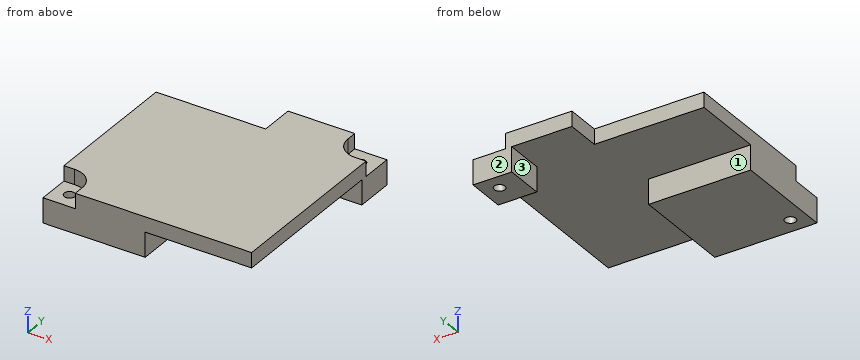
```python
from build123d import *

# Parameters (mm, degrees)
BOSS_EXTRUDE2_DEPTH     = 1.4
SKETCH2_W               = 3.6
SKETCH2_H               = 3.6
SKETCH2_W_2             = 9.5
SKETCH2_H_2             = 9.5
BOSS_EXTRUDE3_DEPTH     = 2.3
CUT_EXTRUDE1_DEPTH      = 14.909349374
CUT_EXTRUDE1_DEPTH_BACK = 14.909349374
SKETCH4_R               = 0.5


with BuildPart() as part:
    # Sketch1 → Boss-Extrude2 (new body)
    with BuildSketch(Plane.XY):
        with BuildLine():
            Line((-6.7, -9.7), (9.7, -9.7))
            Line((9.7, -9.7), (9.7, 6.7))
            Line((9.7, 6.7), (8.7, 6.7))
            ThreePointArc((8.7, 6.7), (7.285786438, 7.285786438), (6.7, 8.7))
            Line((6.7, 8.7), (6.7, 9.7))
            Line((6.7, 9.7), (0.5, 9.7))
            Line((0.5, 9.7), (0.5, 6.5))
            Line((0.5, 6.5), (-9.7, 6.5))
            Line((-9.7, 6.5), (-9.7, -6.7))
            Line((-9.7, -6.7), (-8.7, -6.7))
            ThreePointArc((-8.7, -6.7), (-7.285786438, -7.285786438), (-6.7, -8.7))
            Line((-6.7, -8.7), (-6.7, -9.7))
        make_face()
    extrude(amount=BOSS_EXTRUDE2_DEPTH)

    # Sketch2 → Boss-Extrude3 (add)
    with BuildSketch(Plane(origin=(0, 0, 0), x_dir=(-1, 0, 0), z_dir=(0, 0, -1))):
        with Locations((-7.9, 7.9)):
            Rectangle(SKETCH2_W, SKETCH2_H)
        with Locations((4.95, -4.95)):
            Rectangle(SKETCH2_W_2, SKETCH2_H_2)
    extrude(amount=BOSS_EXTRUDE3_DEPTH)

    # Sketch4 → Cut-Extrude1 (cut, two sides: drawn at the far end of the back side and taken through both)
    with BuildSketch(Plane.XY.offset(-CUT_EXTRUDE1_DEPTH_BACK)):
        with Locations((8.2, 8.2)):
            Circle(SKETCH4_R)
        with Locations((-8.2, -8.2)):
            Circle(SKETCH4_R)
    extrude(amount=CUT_EXTRUDE1_DEPTH + CUT_EXTRUDE1_DEPTH_BACK, mode=Mode.SUBTRACT)


solid = part.part
```
The listing builds one solid part. Answer for the finished solid, in the listing's coordinates (mm). Face numbers are marked on the shaded views. A direction names the side the tool comes from. Coordinates: 2 decimals unless noted, no trailing zeros. Loops run counter-clockwise (first coordinate to the right, second up) from the corner with the lowest first, then second, coordinate; pieces in that order, holes last. Notation, with made-up numbers: (76.5, 36.25) - (81.5, 36.25) arc R9 cw to (81.5, 46.25) - close; hole circle Ø9 at (38, 74). An arc over 180 degrees is marked (long way). Use a Markdown table: item, result. Add a question column.
1) Given pin 1 (1.8 mm diameter, centred on x = -4, z = -1, fed in from +Y); pin 2 (1 mm diameter, centred on y = 5, z = -1.5, fed in from -X); pin 3 (0.9 mm diameter, centred on x = 7.5, y = 8, fed in from +Z); pin 4 (1.5 mm diameter, centred on x = -2.5, z = 1, fed in from +Y), each flat-ended and moving along its own axis, determine where each tip first touches the part or whether it passes through.
2) The part is cut by section C-C, the plane x = 8.2. Give the vertices of the cut face in (y, z).
3) For the marked faces 1, 2 and 3, determine the directions among +Z, -Z, +X, -X, +Y, -Y from which every point of the face is accessible in a straight line to the end or side of a thin tool.
4) The part is cut by section B-B, the plane y = -8.2. Give the vertices of the cut face in (x, z).
5) The part is cut by section A-A, the plane z = -1.2. Give the vertices of the cut face in (x, y), and give its area (3 significant figures).
6) Find the intervals of material crossed by line 1 (Y direction, x = -8.2, z = -1.1); line 2 (Y direction, x = 8.2, z = -0.7), in increasing order.
7) The part is cut by section D-D, the plane z = 0.85. Give the vertices of the cut face in (x, y), and give its area (3 significant figures).
Here are the results:
| question | item | result |
|---|---|---|
| 1 | pin 1 | stops at y = -0.2 |
| 1 | pin 2 | passes through |
| 1 | pin 3 | stops at z = 0 |
| 1 | pin 4 | stops at y = 6.5 |
| 2 | outline | (-9.7, 0) - (6.1, 0) - (6.1, -2.3) - (7.7, -2.3) - (7.7, 0) - (6.76, 0) - (6.76, 1.4) - (-9.7, 1.4) - close; (8.7, -2.3) - (9.7, -2.3) - (9.7, 0) - (8.7, 0) - close |
| 3 | face 1 | -Z, +X, -X, +Y |
| 3 | face 2 | +Z, -Z, +X, -X, +Y |
| 3 | face 3 | -Z, -X, +Y, -Y |
| 4 | outline | (-9.7, -2.3) - (-8.7, -2.3) - (-8.7, 0) - (-9.7, 0) - close; (-7.7, -2.3) - (-0.2, -2.3) - (-0.2, 0) - (9.7, 0) - (9.7, 1.4) - (-6.76, 1.4) - (-6.76, 0) - (-7.7, 0) - close |
| 5 | outline | (-9.7, -9.7) - (-0.2, -9.7) - (-0.2, -0.2) - (-9.7, -0.2) - close; (6.1, 6.1) - (9.7, 6.1) - (9.7, 9.7) - (6.1, 9.7) - close; hole circle Ø1 at (-8.2, -8.2); hole circle Ø1 at (8.2, 8.2) |
| 5 | area | 102 mm^2 |
| 6 | line 1 | y = -9.7 to -8.7, -7.7 to -0.2 |
| 6 | line 2 | y = 6.1 to 7.7, 8.7 to 9.7 |
| 7 | outline | (-9.7, -6.7) - (-8.7, -6.7) arc R2 cw to (-6.7, -8.7) - (-6.7, -9.7) - (9.7, -9.7) - (9.7, 6.7) - (8.7, 6.7) arc R2 cw to (6.7, 8.7) - (6.7, 9.7) - (0.5, 9.7) - (0.5, 6.5) - (-9.7, 6.5) - close |
| 7 | area | 327 mm^2 |
